CAD build for the part. Positions are in the model's coordinates, mm. Face numbers are marked on the shaded views. A direction names the side the tool comes from. Give positions to 0.01 mm unless a question says otherwise; leave off trailing zeros. Loops run counter-clockwise (first coordinate to the right, second up) from the corner with the lowest first, then second, coordinate; pieces in that order, holes last.
Item 1: Probe probe 1 along X at (y, z) = (6, 4.25); probe 2 along Y at (x, z) = (23, 4.5); probe 3 along Y at (x, z) = (12.5, 5.25). List the from-to ranges inside material, lowest first.
Item 2: Mould opens along X. For the marked faces 3, 4, 5 and 6 say: released by +X, released by -X, zero draft, split by the parting line, or undercut.
Item 3: Which spindle directions (+Z, -Z, +X, -X, +Y, -Y) get a long thin tool onto all of the face, cutting with end or side? Do the marked faces 1 and 2. Say none if no direction does.
Item 4: Saw through at A-A on y = 12. Give the cut face in (x, z).
Item 5: Saw through at C-C on z = 4.5. Give the number of separate pieces and of enclosed holes in the cut face, plus the area to 3 significant figures.
Item 6: Drop flat-ended pins along their axis: P1, Ø5.5, axis at x = 12.87, y = 6.63, coming from the -Z side; P2, Ø3.5, axis at x = -36.5, y = 9.5, coming from the +Z side. Give the stop position or say it passes through.
Item 7: Saw through at B-B on x = 24. Give the cut face in (y, z).
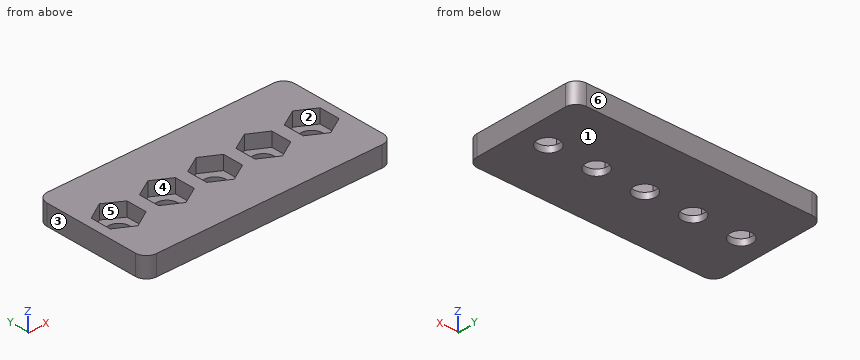
from build123d import *

# Parameters (mm, degrees)
SKETCH3_W           = 79.545894585
SKETCH3_H           = 37.823430605
SKETCH3_R           = 3.5
BOSS_EXTRUDE2_DEPTH = 6.5
SKETCH3_3_R         = 3.5
CUT_EXTRUDE2_DEPTH  = 4.5
FILLET1_R           = 3.5


with BuildPart() as part:
    # Sketch3 → Boss-Extrude2 (new body)
    with BuildSketch(Plane.XY.offset(6.8)):
        with Locations((-2.629280553, 6.684087798)):
            Rectangle(SKETCH3_W, SKETCH3_H)
        with Locations((-33.566454678, 6.627672505)):
            Circle(SKETCH3_R, mode=Mode.SUBTRACT)
        with Locations((-18.129280553, 6.627672505)):
            Circle(SKETCH3_R, mode=Mode.SUBTRACT)
        with Locations((-2.629280553, 6.627672505)):
            Circle(SKETCH3_R, mode=Mode.SUBTRACT)
        with Locations((12.870719447, 6.627672505)):
            Circle(SKETCH3_R, mode=Mode.SUBTRACT)
        with Locations((28.370719447, 6.627672505)):
            Circle(SKETCH3_R, mode=Mode.SUBTRACT)
    extrude(amount=-BOSS_EXTRUDE2_DEPTH)

    # Sketch3<3> → Cut-Extrude2 (cut)
    # profile 1 of 5: a face of its own
    with BuildSketch(Plane.XY.offset(6.8)):
        Polygon((-27.879280553, 9.947436553), (-33.566454678, 13.416303721), (-39.379280553, 9.947436553), (-39.379280553, 3.307908457), (-33.566454678, -0.048128126), (-27.879280553, 3.307908457), (-27.879280553, 6.627672505), align=None)
        with Locations((-33.566454678, 6.627672505)):
            Circle(SKETCH3_3_R, mode=Mode.SUBTRACT)
    # profile 2 of 5: a face of its own
    with BuildSketch(Plane.XY.offset(6.8)):
        Polygon((-23.879280553, 9.947436553), (-23.879280553, 3.307908457), (-18.129280553, -0.01185559), (-12.379280553, 3.307908457), (-12.379280553, 9.947436553), (-18.129280553, 13.267200601), align=None)
        with Locations((-18.129280553, 6.627672505)):
            Circle(SKETCH3_3_R, mode=Mode.SUBTRACT)
    # profile 3 of 5: a face of its own
    with BuildSketch(Plane.XY.offset(6.8)):
        Polygon((34.120719447, 3.307908457), (34.120719447, 9.947436553), (28.370719447, 13.267200601), (22.620719447, 9.947436553), (22.620719447, 6.627672505), (22.620719447, 3.307908457), (28.370719447, -0.01185559), align=None)
        with Locations((28.370719447, 6.627672505)):
            Circle(SKETCH3_3_R, mode=Mode.SUBTRACT)
    # profile 4 of 5: a face of its own
    with BuildSketch(Plane.XY.offset(6.8)):
        Polygon((-8.379280553, 9.947436553), (-8.379280553, 3.307908457), (-2.629280553, -0.01185559), (3.120719447, 3.307908457), (3.120719447, 9.947436553), (-2.629280553, 13.267200601), align=None)
        with Locations((-2.629280553, 6.627672505)):
            Circle(SKETCH3_3_R, mode=Mode.SUBTRACT)
    # profile 5 of 5: a face of its own
    with BuildSketch(Plane.XY.offset(6.8)):
        Polygon((18.620719447, 3.307908457), (18.620719447, 9.947436553), (12.870719447, 13.267200601), (7.120719447, 9.947436553), (7.120719447, 3.307908457), (12.870719447, -0.01185559), align=None)
        with Locations((12.870719447, 6.627672505)):
            Circle(SKETCH3_3_R, mode=Mode.SUBTRACT)
    extrude(amount=-CUT_EXTRUDE2_DEPTH, mode=Mode.SUBTRACT)

    # Fillet1
    fillet1_edges = [part.edges().sort_by_distance(p)[0] for p in [
        (-42.402227845, 25.5958031, 3.55),
        (37.14366674, 25.5958031, 3.55),
        (37.14366674, -12.227627505, 3.55),
        (-42.402227845, -12.227627505, 3.55),
    ]]
    fillet(fillet1_edges, radius=FILLET1_R)


solid = part.part
Results below:
1. probe 1: x = -42.4 to -39.38, -27.88 to -23.88, -12.38 to -8.38, 3.12 to 7.12, 18.62 to 22.62, 34.12 to 37.14
1. probe 2: y = -12.23 to 3.09, 10.17 to 25.6
1. probe 3: y = -12.23 to 0.2, 13.05 to 25.6
2. face 3: released by -X
2. face 4: undercut
2. face 5: undercut
2. face 6: zero draft
3. face 1: -Z, +X, -X, +Y, -Y
3. face 2: +Z
4. outline: (-42.4, 0.3) - (37.14, 0.3) - (37.14, 6.8) - (30.57, 6.8) - (30.57, 2.3) - (26.18, 2.3) - (26.18, 6.8) - (15.07, 6.8) - (15.07, 2.3) - (10.68, 2.3) - (10.68, 6.8) - (-0.43, 6.8) - (-0.43, 2.3) - (-4.82, 2.3) - (-4.82, 6.8) - (-15.93, 6.8) - (-15.93, 2.3) - (-20.32, 2.3) - (-20.32, 6.8) - (-31.24, 6.8) - (-31.24, 2.3) - (-35.94, 2.3) - (-35.94, 6.8) - (-42.4, 6.8) - close
5. separate pieces: 1
5. enclosed holes: 5
5. area: 2,420 mm2
6. P1: passes through
6. P2: stops at z = 2.3
7. outline: (-12.23, 0.3) - (25.6, 0.3) - (25.6, 6.8) - (10.74, 6.8) - (10.74, 2.3) - (2.51, 2.3) - (2.51, 6.8) - (-12.23, 6.8) - close
